Could you check a few things on this model? Use its own coordinates, in mm. A direction names the side the tool comes from. Give positions to 0.01 mm unless a question says otherwise; leave off trailing zeros. Loops run counter-clockwise (first coordinate to the right, second up) from the corner with the lowest first, then second, coordinate; pieces in that order, holes last. Notation, with made-up numbers: M 85.5,-29.75 L 119.5,-29.75 A29 cw 119.5,3.25 Z; hole C -13.75,52.25 d8. An arc over 180 degrees is marked long. Use a Markdown table: item, result. Add a question column.
1) Will these pins go through, and if not, where does the flat tip stop? pin 1 Ø1 at (x, y) = (7.5, -15.5) entering from -Z; pin 2 Ø1.5 at (x, y) = (-6.5, -17.5) entering from -Z; pin 3 Ø5 at (x, y) = (-6, -11.5) entering from +Z.
2) Which directions (+Z, -Z, +X, -X, +Y, -Y) give clear straight access to the entire face, cutting with the end or side of a thin tool? Please do faces 1 (the flat face through (-6, -0.965, -25)), 2 (the flat face through (7.2, 3, -29.6)), 3 (the flat face through (7.206, -2.808, -34.148)), 4 (the cylindrical face through (6.19, -20.24, -29.16)).
3) We'd pull the mould along X, two halves only. Please class faces 5 (the cylindrical face through (-9.137, -0.476, -25.814)), 6 (the flat face through (26.472, -2, -21)), 7 (the flat face through (6.32, -6.45, -25.15)): +X half, -X half, draft (parallel to the pull), parting line (faces both ways), or undercut.
4) Suppose I cut it at A-A on x = -0.5. List the corners of the cut face in (y, z) for me, and give its area (3 significant figures).
5) If I drill on line 1 along X through (y, z) = (-0.25, -19); line 2 along Z through (x, y) = (12.5, -0.25); line 3 along Z through (x, y) = (-0.5, -6), over which ranges is the centre line in solid material (lowest first)? Write a range as [from, to].
6) Suppose I cut it at C-C on y = -17.75. List the corners of the cut face in (x, z) for me, and give its area (3 significant figures).
7) Suppose I cut it at D-D on z = -21.5. List the corners of the cut face in (x, y) for me, and give its area (3 significant figures).
8) Suppose I cut it at B-B on z = -9.5. List the corners of the cut face in (x, y) for me.
```python
from build123d import *

# Parameters (mm, degrees)
F0_W     = 40
F0_H     = 40
F0_R     = 2.8088717
F0_R_2   = 2.8088682771
F1_DEPTH = 1
F3_DEPTH = 40
F4_DEPTH = 2
F5_DEPTH = 18.288
F5_TAPER = -20
F6_DEPTH = 9.0678
F6_TAPER = -20
F7_START = 0.9652
F7_DEPTH = 11.557


with BuildPart() as f1:
    # F0 (on Front) → F1 (new body)
    with BuildSketch(Plane.XZ):
        with Locations((6.4715254307, -8.0715133995)):
            Rectangle(F0_W, F0_H)
        with BuildLine():
            Line((-5.4296746384, -19.3524439185), (-5.4296746384, 3.8296866696))
            Line((-5.4296746384, 3.8296866696), (18.3727254998, 3.8296866696))
            Line((18.3727254998, 3.8296866696), (18.3727254998, -19.3524439185))
            ThreePointArc((18.3727254998, -19.3524439185), (23.524954992, -18.6877403838), (26.3123971307, -23.0715133995))
            ThreePointArc((26.3123971307, -23.0715133995), (19.8237237716, -27.6233029935), (17.7524559497, -19.9727134686))
            Line((17.7524559497, -19.9727134686), (-4.8094050884, -19.9727134686))
            ThreePointArc((-4.8094050884, -19.9727134686), (-3.9766849753, -21.4237117404), (-3.6876028693, -23.0715133995))
            ThreePointArc((-3.6876028693, -23.0715133995), (-12.912247585, -25.1249429608), (-5.4296746384, -19.3524439185))
        make_face(mode=Mode.SUBTRACT)
        with Locations((-8.5284745693, 6.9284866005)):
            Circle(F0_R, mode=Mode.SUBTRACT)
        with Locations((21.4715254307, 6.9284866005)):
            Circle(F0_R_2, mode=Mode.SUBTRACT)
        with BuildLine():
            Line((-5.4296746384, -19.9727134686), (-5.4296746384, -19.3524439185))
            ThreePointArc((-5.4296746384, -19.3524439185), (-12.912247585, -25.1249429608), (-3.6876028693, -23.0715133995))
            ThreePointArc((-3.6876028693, -23.0715133995), (-3.9766849753, -21.4237117404), (-4.8094050884, -19.9727134686))
            Line((-4.8094050884, -19.9727134686), (-5.4296746384, -19.9727134686))
        make_face()
        with Locations((-8.5284745693, -23.0715133995)):
            Circle(F0_R, mode=Mode.SUBTRACT)
        with BuildLine():
            ThreePointArc((26.3123971307, -23.0715133995), (23.524954992, -18.6877403838), (18.3727254998, -19.3524439185))
            Line((18.3727254998, -19.3524439185), (18.3727254998, -19.9727134686))
            Line((18.3727254998, -19.9727134686), (17.7524559497, -19.9727134686))
            ThreePointArc((17.7524559497, -19.9727134686), (19.8237237716, -27.6233029935), (26.3123971307, -23.0715133995))
        make_face()
        with Locations((21.4715254307, -23.0715133995)):
            Circle(F0_R, mode=Mode.SUBTRACT)
    extrude(amount=F1_DEPTH)

    # F2 (on face) → F3 (join)
    with BuildSketch(Plane(origin=(-13.5284745693, 0, 0), x_dir=(0, -1, 0), z_dir=(-1, 0, 0))):
        with BuildLine():
            Line((12.3116524944, -33.2211739971), (-6.9665359333, -35.1002924144))
            Line((-6.9665359333, -35.1002924144), (-6.8581130742, -36.2126205614))
            Line((-6.8581130742, -36.2126205614), (12.4200753535, -34.333502144))
            ThreePointArc((12.4200753535, -34.333502144), (20.3048000078, -29.0359972653), (20.2130647017, -19.5373644454))
            Line((20.2130647017, -19.5373644454), (12.0343582979, -4.7106706036))
            Line((12.0343582979, -4.7106706036), (1.9645202799, 12.4930484239))
            Line((1.9645202799, 12.4930484239), (0, 12.4930484239))
            Line((0, 12.4930484239), (0, 11.9284866005))
            Line((0, 11.9284866005), (1, 11.9284866005))
            Line((1, 11.9284866005), (11.0626462847, -5.2629457787))
            Line((11.0626462847, -5.2629457787), (19.2344762678, -20.0771737634))
            ThreePointArc((19.2344762678, -20.0771737634), (19.3159684051, -28.5151887743), (12.3116524944, -33.2211739971))
        make_face()
        Polygon((1, -19.8451913893), (1, -28.0715133995), (4.8349229619, -27.460442856), (6.5377627002, -26.0303480879), (6.3641844317, -24.2495797575), align=None)
        Polygon((-6.9665359333, -31.1145037413), (1, -28.0715133995), (0, -28.0715133995), (0, -26.7824456096), (-6.9665359333, -29.9953967333), align=None)
    extrude(amount=-F3_DEPTH)

    # F2 (on face) → F4 (join)
    with BuildSketch(Plane(origin=(-13.5284745693, 0, 0), x_dir=(0, -1, 0), z_dir=(-1, 0, 0))):
        with BuildLine():
            Line((4.8349229619, -27.460442856), (1, -28.0715133995))
            Line((1, -28.0715133995), (-6.9665359333, -31.1145037413))
            Line((-6.9665359333, -31.1145037413), (-6.9665359333, -35.1002924144))
            Line((-6.9665359333, -35.1002924144), (12.3116524944, -33.2211739971))
            ThreePointArc((12.3116524944, -33.2211739971), (19.3159684051, -28.5151887743), (19.2344762678, -20.0771737634))
            Line((19.2344762678, -20.0771737634), (11.0626462847, -5.2629457787))
            Line((11.0626462847, -5.2629457787), (1, 11.9284866005))
            Line((1, 11.9284866005), (1, -19.8451913893))
            Line((1, -19.8451913893), (6.3641844317, -24.2495797575))
            Line((6.3641844317, -24.2495797575), (6.5377627002, -26.0303480879))
            Line((6.5377627002, -26.0303480879), (4.8349229619, -27.460442856))
        make_face()
    extrude(amount=-F4_DEPTH)

    # F0 (on Front) → F5 (cut)
    with BuildSketch(Plane.XZ):
        with Locations((21.4715254307, 6.9284866005)):
            Circle(F0_R_2)
    extrude(amount=F5_DEPTH, taper=F5_TAPER, mode=Mode.SUBTRACT)

    # F0 (on Front) → F6 (cut)
    with BuildSketch(Plane.XZ):
        with Locations((-8.5284745693, 6.9284866005)):
            Circle(F0_R)
    extrude(amount=F6_DEPTH, taper=F6_TAPER, mode=Mode.SUBTRACT)

    # F0 (on Front) → F7 (cut)
    with BuildSketch(Plane.XZ.offset(F7_START)):
        with BuildLine():
            ThreePointArc((26.3123971307, -23.0715133995), (23.524954992, -18.6877403838), (18.3727254998, -19.3524439185))
            Line((18.3727254998, -19.3524439185), (18.3727254998, -19.9727134686))
            Line((18.3727254998, -19.9727134686), (17.7524559497, -19.9727134686))
            ThreePointArc((17.7524559497, -19.9727134686), (19.8237237716, -27.6233029935), (26.3123971307, -23.0715133995))
        make_face()
        with Locations((21.4715254307, -23.0715133995)):
            Circle(F0_R, mode=Mode.SUBTRACT)
        with BuildLine():
            Line((-5.4296746384, -19.9727134686), (-5.4296746384, -19.3524439185))
            ThreePointArc((-5.4296746384, -19.3524439185), (-12.912247585, -25.1249429608), (-3.6876028693, -23.0715133995))
            ThreePointArc((-3.6876028693, -23.0715133995), (-3.9766849753, -21.4237117404), (-4.8094050884, -19.9727134686))
            Line((-4.8094050884, -19.9727134686), (-5.4296746384, -19.9727134686))
        make_face()
        with Locations((-8.5284745693, -23.0715133995)):
            Circle(F0_R, mode=Mode.SUBTRACT)
        with Locations((21.4715254307, -23.0715133995)):
            Circle(F0_R)
        with Locations((-8.5284745693, -23.0715133995)):
            Circle(F0_R)
    extrude(amount=F7_DEPTH, mode=Mode.SUBTRACT)


solid = f1.part
```
Answer block:
| question | item | result |
|---|---|---|
| 1 | pin 1 | stops at z = -33.73 |
| 1 | pin 2 | stops at z = -32.86 |
| 1 | pin 3 | stops at z = 0.47 |
| 2 | face 1 | none |
| 2 | face 2 | +X |
| 2 | face 3 | +X, +Y |
| 2 | face 4 | +X, -X, -Y |
| 3 | face 5 | undercut |
| 3 | face 6 | +X half |
| 3 | face 7 | draft |
| 4 | outline | M -20.21,-19.54 A10.01 ccw -12.42,-34.33 L 6.86,-36.21 L 6.97,-35.1 L -12.31,-33.22 A8.89 cw -19.23,-20.08 L -11.06,-5.26 L -1,11.93 L -1,3.83 L 0,3.83 L 0,12.49 L -1.96,12.49 L -12.03,-4.71 Z; M -6.54,-26.03 L -4.83,-27.46 L -1,-28.07 L 6.97,-31.11 L 6.97,-30 L 0,-26.78 L 0,-19.97 L -1,-19.97 L -1,-19.85 L -6.36,-24.25 Z |
| 4 | area | 140 mm^2 |
| 5 | line 1 | x = [-13.53, -5.43], [18.37, 26.47] |
| 5 | line 2 | z = [-35.52, -34.4], [-28.36, -19.97], [3.83, 12.49] |
| 5 | line 3 | z = [-34.96, -33.84], [-26.48, -23.95], [3.39, 5.6] |
| 6 | outline | M -13.53,-32.15 L 26.47,-32.15 L 26.47,-30.65 L -11.53,-30.65 L -11.53,-17.39 L 26.47,-17.39 L 26.47,-15.07 L -13.53,-15.07 Z |
| 6 | area | 179 mm^2 |
| 7 | outline | M -13.53,-21.04 L 26.47,-21.04 L 26.47,-19.86 L -11.53,-19.86 L -11.53,-12.52 L -13.11,-12.52 L -13.11,-0.97 L -10.86,-0.97 L -10.86,0 L -13.53,0 Z; M -6.2,-0.97 L -3.95,-0.97 L -3.95,-3.02 L 16.89,-3.02 L 16.89,-0.97 L 19.14,-0.97 L 19.14,0 L -6.2,0 Z; M 23.8,-0.97 L 26.05,-0.97 L 26.05,-3.02 L 26.47,-3.02 L 26.47,0 L 23.8,0 Z |
| 7 | area | 140 mm^2 |
| 8 | outline | M -13.53,-14.68 L 26.47,-14.68 L 26.47,-13.4 L -11.53,-13.4 L -11.53,-1 L -5.43,-1 L -5.43,0 L -13.53,0 Z; M 18.37,-1 L 26.47,-1 L 26.47,0 L 18.37,0 Z |
